For this review, take the finished solid that the model builds, in its own axes (mm). Face numbers are marked on the shaded views. A direction names the side the tool comes from. Give positions to 0.01 mm unless a question says otherwise; leave off trailing zeros. Loops run counter-clockwise (first coordinate to the right, second up) from the corner with the lowest first, then second, coordinate; pieces in that order, holes last.
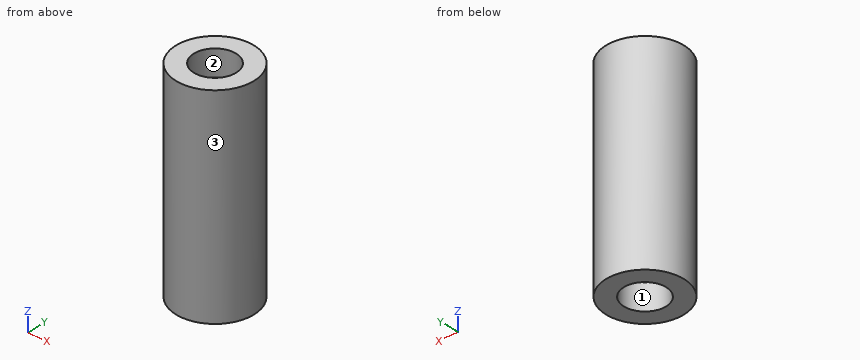
```python
from build123d import *

# Parameters (mm, degrees)
F1_R     = 9.525
F2_DEPTH = 50.8
F5_D     = 4.2
F6_D     = 10.31748
F6_DEPTH = 6.35
F6_TIP   = 3.0996837098
F8_D     = 10.31748
F8_DEPTH = 6.35
F8_TIP   = 3.0996837098


with BuildPart() as f2:
    # F1 (on Top) → F2 (new body, through all)
    with BuildSketch(Plane.XY):
        Circle(F1_R)
    extrude(amount=-F2_DEPTH)

    # F5 (through all)
    with Locations(Plane.XY):
        with Locations((0, 0)):
            Hole(F5_D / 2)

    # F6
    with Locations(Plane(origin=(0, 0, -50.8), x_dir=(1, 0, 0), z_dir=(0, 0, -1))):
        with Locations((0, 0)):
            Hole(F6_D / 2, depth=F6_DEPTH)
            with Locations((0, 0, -(F6_DEPTH + F6_TIP / 2))):  # 118° drill point
                Cone(0, F6_D / 2, F6_TIP, mode=Mode.SUBTRACT)

    # F8
    with Locations(Plane.XY):
        with Locations((0, 0)):
            Hole(F8_D / 2, depth=F8_DEPTH)
            with Locations((0, 0, -(F8_DEPTH + F8_TIP / 2))):  # 118° drill point
                Cone(0, F8_D / 2, F8_TIP, mode=Mode.SUBTRACT)


solid = f2.part
```
Q1. For pin 1 Ø5 at (y, z) = (5, -43) entering from +X; pin 2 Ø1.5 at (y, z) = (3, -29.5) entering from -X; pin 3 Ø8 at (x, z) = (-6, -18) entering from -Y, all flat-tipped, find the tip position at first contact; note any pin that passes through.
Answers:
pin 1: stops at x = 9.19
pin 2: stops at x = -9.26
pin 3: stops at y = -9.31
Q2. Consider section D-D on x = -7.75. Give the boundary of the cut face in (y, z).
Answers:
outline: (-5.54, -50.8) - (5.54, -50.8) - (5.54, 0) - (-5.54, 0) - close
Q3. Consider section C-C on z = -26. Give the boundary of the cut face in (x, y) (3 decimals), plus the area to 3 significant figures.
Answers:
outline: circle Ø19.05 at (0, 0); hole circle Ø4.2 at (0, 0)
area: 271 mm2
Q4. Machinability: for the marked faces 1, 2 and 3, which of the approach directions +Z, -Z, +X, -X, +Y, -Y give a long, thin tool a straight path to every point of the face, cutting with its end or side? Answer none if there is none.
Answers:
face 1: -Z
face 2: +Z
face 3: +Z, -Z
Q5. Consider section A-A on y = 0. Give the boundary of the cut face in (x, z) (3 decimals), plus the area to 3 significant figures.
Answers:
outline: (-9.525, -50.8) - (-5.159, -50.8) - (-5.159, -44.45) - (-2.1, -42.612) - (-2.1, -8.188) - (-5.159, -6.35) - (-5.159, 0) - (-9.525, 0) - close; (2.1, -42.612) - (5.159, -44.45) - (5.159, -50.8) - (9.525, -50.8) - (9.525, 0) - (5.159, 0) - (5.159, -6.35) - (2.1, -8.188) - close
area: 665 mm2
Q6. For probe 1 along Y at (x, z) = (0, -46) (3 decimals); probe 2 along Y at (x, z) = (0, -30.5) (3 decimals); probe 3 along X at (y, z) = (0.5, -45), list the stretches that pass through material, from the lowest coordinate up.
Answers:
probe 1: y = -9.525 to -5.159, 5.159 to 9.525
probe 2: y = -9.525 to -2.1, 2.1 to 9.525
probe 3: x = -9.51 to -5.13, 5.13 to 9.51
